Job drawing, mm, ordinate dimensions from the low corner. One solid piece. A direction names the side the tool comes from. Round coordinates to 2 decimals unless told otherwise and drop trailing zeros. Loops run counter-clockwise (first coordinate to the right, second up) from the corner with the lowest first, then second, coordinate; pieces in that order, holes last.
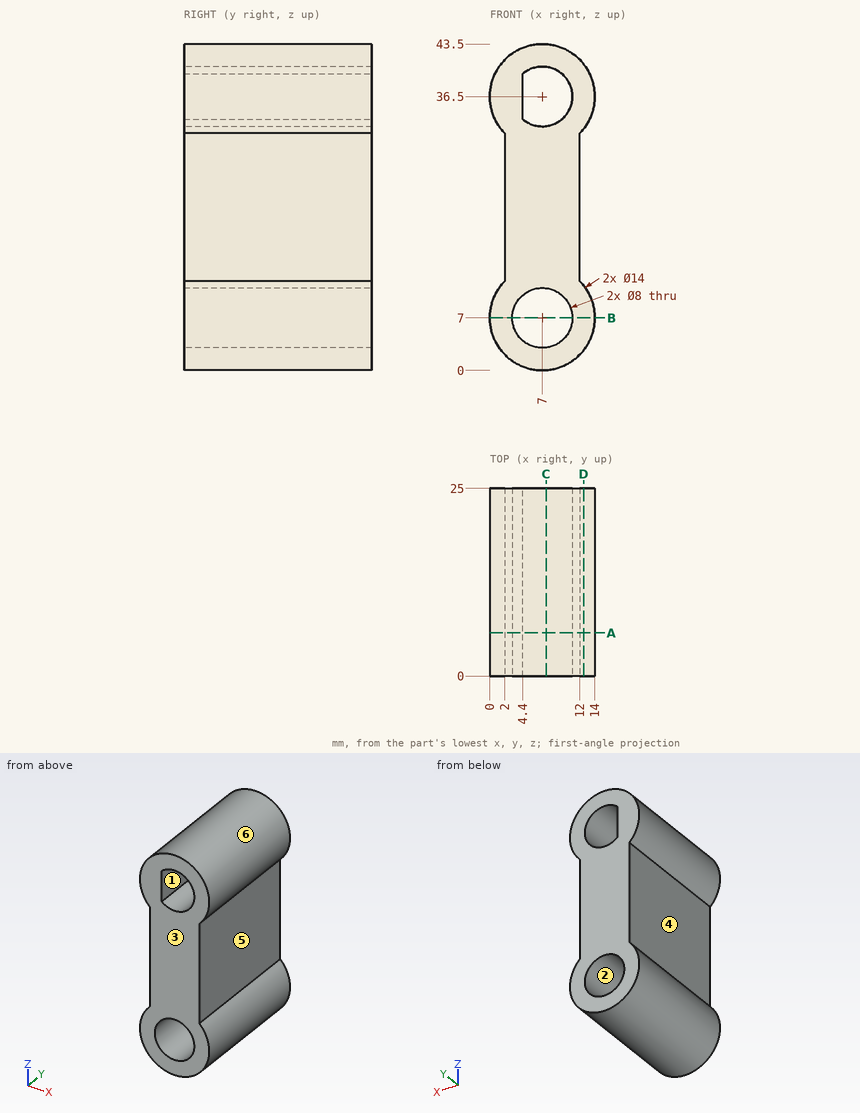
Item 1: Two-plate mould, pull along Z, no slides. Class the marked faces 1, 2 and 3: released by +Z, released by -Z, zero draft, split by the parting line, or undercut.
Answers follow:
face 1: undercut
face 2: undercut
face 3: zero draft
Item 2: Cut at C-C, the plane x = 7.5. Give the cut face in (y, z), plus the area to 3 significant figures.
Answers follow:
outline: (0, 0.02) - (25, 0.02) - (25, 3.03) - (0, 3.03) - close; (0, 10.97) - (25, 10.97) - (25, 32.53) - (0, 32.53) - close; (0, 40.47) - (25, 40.47) - (25, 43.48) - (0, 43.48) - close
area: 690 mm2
Item 3: Cut at A-A, the plane y = 5.75. Give the cut face in (x, z), plus the area to 3 significant figures.
Answers follow:
outline: (2, 11.9) arc R7 ccw (long way) to (12, 11.9) - (12, 31.6) arc R7 ccw (long way) to (2, 31.6) - close; hole circle Ø8 at (7, 7); hole (4.4, 33.46) arc R4 ccw (long way) to (4.4, 39.54) - close
area: 381 mm2
Item 4: Flat gauge pins, fed straight in: P1, Ø8, axis at y = 4.5, z = 28, coming from the +X side; P2, Ø3, axis at y = 16.5, z = 27, coming from the -X side; P3, Ø5, axis at x = 10.5, z = 38.5, coming from the -Y side. Where does each tip first touch, or does it go through?
Answers follow:
P1: stops at x = 12.36
P2: stops at x = 2
P3: stops at y = 0
Item 5: Cut at D-D, the plane x = 12.5. Give the cut face in (y, z), plus the area to 3 significant figures.
Answers follow:
outline: (0, 2.67) - (25, 2.67) - (25, 11.33) - (0, 11.33) - close; (0, 32.17) - (25, 32.17) - (25, 40.83) - (0, 40.83) - close
area: 433 mm2
Item 6: 3-axis set-ups, long thin cutter, end or side, ignore diameter. For the marked faces 4, 5 and 6: which of +Z, -Z, +X, -X, +Y, -Y reach the whole face in a straight line?
Answers follow:
face 4: -X, +Y, -Y
face 5: +X, +Y, -Y
face 6: +Y, -Y
Item 7: Probe line 1 (X direction, y = 10.5, z = 7); line 2 (Z direction, x = 10.5, y = 18.75); line 3 (Z direction, x = 8, y = 5.25). List the from-to ranges inside material, lowest first.
Answers follow:
line 1: x = 0 to 3, 11 to 14
line 2: z = 0.94 to 5.06, 8.94 to 34.56, 38.44 to 42.56
line 3: z = 0.07 to 3.13, 10.87 to 32.63, 40.37 to 43.43
Item 8: Cut at B-B, the plane z = 7. Give the cut face in (x, y).
Answers follow:
outline: (0, 0) - (3, 0) - (3, 25) - (0, 25) - close; (11, 0) - (14, 0) - (14, 25) - (11, 25) - close
